Part model, mm, in its own coordinate system. A direction names the side the tool comes from. Coordinates: 2 decimals unless noted, no trailing zeros. Loops run counter-clockwise (first coordinate to the right, second up) from the corner with the lowest first, then second, coordinate; pieces in that order, holes last.
Autodesk Inventor part; units mm, degrees
ref_plane "YZ Plane" through (0, 0, 0) normal (1, 0, 0) x (0, 1, 0)
ref_plane "XZ Plane" through (0, 0, 0) normal (0, 1, 0) x (-1, 0, 0)
ref_plane "XY Plane" through (0, 0, 0) normal (0, 0, 1) x (1, 0, 0)
sketch "Sketch1" plane through (0, 0, 0) normal (0, 0, 1) x (1, 0, 0)
  line L0 (-28.5, -28.5) -> (28.5, -28.5)
  line L1 (28.5, -28.5) -> (28.5, 28.5)
  line L2 (28.5, 28.5) -> (-28.5, 28.5)
  line L3 (-28.5, 28.5) -> (-28.5, -28.5)
  line L4 (-28.5, -28.5) -> (28.5, 28.5) construction
  line L5 (28.5, -28.5) -> (-28.5, 28.5) construction
  point P0 (0, 0)
  dimension "d0" = 57
  dimension "d1" = 57
extrude "Extrusion1" add sketch "Sketch1" against normal blind 2.921
sketch "Sketch2" plane through (0, 0, 0) normal (0, 0, 1) x (1, 0, 0)
  line L0 (-10.0551, 28.5) -> (-9.5, 28.5)
  line L1 (-9.5, 28.5) -> (-9.5, 25.5)
  line L2 (-9.5, 25.5) -> (9.5, 25.5)
  line L3 (9.5, 25.5) -> (9.5, 28.5)
  line L4 (-9.5, 28.5) -> (9.5, 28.5)
  line L5 (-9.5, -28.5) -> (9.5, -28.5)
  line L6 (9.5, -28.5) -> (9.5, -25.5)
  line L7 (9.5, -25.5) -> (-9.5, -25.5)
  line L8 (-9.5, -25.5) -> (-9.5, -28.5)
  line L9 (-28.5, 9.5) -> (-25.5, 9.5)
  line L10 (-25.5, 9.5) -> (-25.5, -9.5)
  line L11 (-25.5, -9.5) -> (-28.5, -9.5)
  line L12 (-28.5, -9.5) -> (-28.5, 9.5)
  line L13 (28.5, 9.5) -> (25.5, 9.5)
  line L14 (25.5, 9.5) -> (25.5, -9.5)
  line L15 (25.5, -9.5) -> (28.5, -9.5)
  line L16 (28.5, -9.5) -> (28.5, 9.5)
  line L17 (28.5, -28.5) -> (28.5, 28.5)
  line L18 (-28.5, 28.5) -> (-28.5, -28.5)
  line L19 (-28.5, -28.5) -> (28.5, -28.5)
  line L20 (28.5, 28.5) -> (-28.5, 28.5)
  line L21 (-28.5, 28.5) -> (-28.5, -28.5)
  dimension "d4" = 3
  dimension "d5" = 19
  dimension "d17" = 19
  dimension "d18" = 3
  dimension "d19" = 3
  dimension "d20" = 19
  dimension "d34" = 3
  dimension "d35" = 19
  dimension "d47" = 19
  dimension "d48" = 19
  dimension "d49" = 19
  dimension "d50" = 19
  dimension "d51" = 19
  dimension "d52" = 19
  dimension "d54" = 19
  dimension "d55" = 19
extrude "Extrusion3" cut sketch "Sketch2" against normal blind 25.4 contours L4 L3 L2 L1 | L9 L10 L11 L12 | L16 L15 L14 L13 | L8 L7 L6 L5
hole "Hole1" at (0, 0, 0) direction (0, 0, -1) diameter 25.4 end through all
equation "\"d1\" = d0"
equation "\"d17\" = d5"
equation "\"d18\" = d4"
equation "\"d19\" = d4"
equation "\"d20\" = d5"
equation "\"d34\" = d4"
equation "\"d35\" = d5"
equation "\"d47\" = -0.5 * d5 + 0.5 * d0"
equation "\"d49\" = d47"
equation "\"d50\" = d47"
equation "\"d51\" = d47"
equation "\"d23\" = 0.5 * d0"
equation "\"d53\" = 0.5 * d0"
properties part number "Side A"
Q1. Probe line 1 (X direction, y = 0, z = -2.2); line 2 (Y direction, x = -10, z = -1.85). List the from-to ranges inside material, lowest first.
Q2. Drop flat-ended pins along their axis: P1, Ø1, axis at y = -1, z = -2, coming from the +X side; P2, Ø0.9, axis at x = 3.5, z = -1.5, coming from the -Y side; P3, Ø1.5, axis at y = 8.5, z = -0.5, coming from the -X side. Give the stop position or say it passes through.
Q3. Saw through at A-A (x = 0). List the corners of the cut face in (y, z).
Q4. Tool access for faces 5 (the flat face through (25.5, 0, -1)), 6 (the flat face through (-27, 9.5, -1)), 7 (the flat face through (-19, -28.5, -1)), 8 (the flat face through (-9.5, 27, -1)): list every direction of +Z, -Z, +X, -X, +Y, -Y with a clear straight run to the whole face (end or side of a thin tool).
Q5. Saw through at C-C (z = -1.1). List the corners of the cut face in (x, y).
Q6. Mould opens along X. For faces 1 (the flat face through (28.5, -19, -1)), 2 (the flat face through (19, 28.5, -1)), 3 (the flat face through (0, 25.5, -1)), 4 (the flat face through (9.5, -27, -1)) say: released by +X, released by -X, zero draft, split by the parting line, or undercut.
Checked values:
1. line 1: x = -25.5 to -12.7, 12.7 to 25.5
1. line 2: y = -28.5 to -7.83, 7.83 to 28.5
2. P1: stops at x = 25.5
2. P2: stops at y = -25.5
2. P3: stops at x = -25.5
3. outline: (-25.5, -2.92) - (-12.7, -2.92) - (-12.7, 0) - (-25.5, 0) - close; (12.7, -2.92) - (25.5, -2.92) - (25.5, 0) - (12.7, 0) - close
4. face 5: +Z, -Z, +X
4. face 6: +Z, -Z, -X
4. face 7: +Z, -Z, +X, -X, -Y
4. face 8: +Z, -Z, +Y
5. outline: (-28.5, -28.5) - (-9.5, -28.5) - (-9.5, -25.5) - (9.5, -25.5) - (9.5, -28.5) - (28.5, -28.5) - (28.5, -9.5) - (25.5, -9.5) - (25.5, 9.5) - (28.5, 9.5) - (28.5, 28.5) - (9.5, 28.5) - (9.5, 25.5) - (-9.5, 25.5) - (-9.5, 28.5) - (-28.5, 28.5) - (-28.5, 9.5) - (-25.5, 9.5) - (-25.5, -9.5) - (-28.5, -9.5) - close; hole circle Ø25.4 at (0, 0)
6. face 1: released by +X
6. face 2: zero draft
6. face 3: undercut
6. face 4: undercut
